from build123d import *

# Parameters (mm, degrees)
SKETCH5_R           = 3.175
BOSS_EXTRUDE3_DEPTH = 88.9
BOSS_EXTRUDE4_DEPTH = 3.96875
SKETCH8_OUTSIDE_W   = 357.164
SKETCH8_OUTSIDE_H   = 358.884
SKETCH8_OUTSIDE_R   = 5.55625
CUT_EXTRUDE3_DEPTH  = 93.86875
CUT_EXTRUDE3_TAPER  = 60
CUT_EXTRUDE4_DEPTH  = 0.254
CIRPATTERN1_COUNT   = 3


with BuildPart() as part:
    # Sketch5 → Boss-Extrude3 (new body)
    with BuildSketch(Plane(origin=(46.434375, 0, 0), x_dir=(0, 0, -1), z_dir=(1, 0, 0))):
        Circle(SKETCH5_R)
    extrude(amount=-BOSS_EXTRUDE3_DEPTH)

    # Sketch11 → Revolve1 (revolve)
    with BuildSketch(Plane.XY):
        Polygon((-42.465625, 3.175), (-42.465625, 0), (30.559375, 0), (27.384375, 3.175), align=None)
    revolve(axis=Axis((-42.465625, 0, 0), (1, 0, 0)))

    # Sketch6 → Boss-Extrude4 (add)
    with BuildSketch(Plane.ZY.offset(42.465625)):
        Polygon((5.55625, 3.207902433), (0, 6.415804866), (-5.55625, 3.207902433), (-5.55625, -3.207902433), (0, -6.415804866), (5.55625, -3.207902433), align=None)
    extrude(amount=BOSS_EXTRUDE4_DEPTH)

    # Sketch8 outside → Cut-Extrude3 (cut, through all)
    with BuildSketch(Plane.ZY.offset(46.434375)):
        Rectangle(SKETCH8_OUTSIDE_W, SKETCH8_OUTSIDE_H)
        Circle(SKETCH8_OUTSIDE_R, mode=Mode.SUBTRACT)
    extrude(amount=-CUT_EXTRUDE3_DEPTH, taper=CUT_EXTRUDE3_TAPER, mode=Mode.SUBTRACT)

    # Sketch12 → Cut-Extrude4 (cut)
    with BuildSketch(Plane.ZY.offset(46.434375)):
        with BuildLine():
            Line((0.1666875, 4.2783125), (0.1666875, 2.3891875))
            ThreePointArc((0.1666875, 2.3891875), (0, 2.2225), (-0.1666875, 2.3891875))
            Line((-0.1666875, 2.3891875), (-0.1666875, 4.2783125))
            ThreePointArc((-0.1666875, 4.2783125), (0, 4.445), (0.1666875, 4.2783125))
        make_face()
    cut_extrude4 = extrude(amount=-CUT_EXTRUDE4_DEPTH, mode=Mode.SUBTRACT)

    # CirPattern1: Cut-Extrude4 ×3 about axis
    cirpattern1_axis = Axis((0, 0, 0), (1, 0, 0))
    for i in range(1, CIRPATTERN1_COUNT):
        add(cut_extrude4.rotate(cirpattern1_axis, i * 360 / CIRPATTERN1_COUNT), mode=Mode.SUBTRACT)


solid = part.part
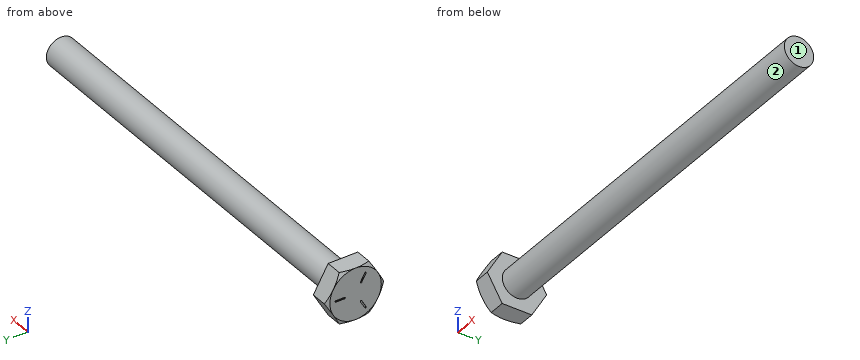
Geometry check sheet. Reference: the model listing, model coordinates, mm. Face numbers are marked on the shaded views. A direction names the side the tool comes from. Round coordinates to 2 decimals unless told otherwise and drop trailing zeros. Order: outer loops, then holes, each group sorted by start corner. A loop starts at its lowest first (then second) coordinate and runs counter-clockwise, first axis right, second up. Notation, with made-up numbers: M 85.5,8.25 L 96.5,8.25 A31 cw 96.5,41.25 Z; hole C 89,9.25 d5. An arc over 180 degrees is marked long. Answer in a Markdown table with one row per item. Add a question column.
Item 1: Set-up check for the marked faces 1 and 2: record each of +Z, -Z, +X, -X, +Y, -Y from which the full face is reachable in a straight line by a thin tool's end or side.
Item 2: Depth check by flat-ended pin: pin 1 Ø5 at (x, y) = (-23.5, -4) entering from -Z; pin 2 Ø1 at (x, z) = (20.5, 2.5) entering from -Y; pin 3 Ø4 at (x, y) = (-27, 1) entering from +Z (3 decimals). Enter the tip coordinate at first touch or a pass-through.
Item 3: Material ranges on L1, parallel to Y at x = -32.5, z = -0.25; L2, parallel to X at y = -4.75, z = 1.75; L3, parallel to Z at x = -40, y = 0 (3 decimals), recorded low to high. Write a range as [from, to].
Item 4: Sectioned sample at A-A, the plane x = 21. Enter the section's corners in (y, z) (3 decimals), plus the area to 3 significant figures.
Filled in:
| question | item | result |
|---|---|---|
| 1 | face 1 | +Z, -Z, +X, +Y, -Y |
| 1 | face 2 | +X |
| 2 | pin 1 | stops at z = -2.8 |
| 2 | pin 2 | stops at y = -2.47 |
| 2 | pin 3 | stops at z = 3.175 |
| 3 | L1 | y = [-3.17, 3.17] |
| 3 | L2 | x = [-46.43, -42.47] |
| 3 | L3 | z = [-3.175, 3.175] |
| 4 | outline | C 0,0 d6.35 |
| 4 | area | 31.7 mm² |
